```python
from build123d import *

# Parameters (mm, degrees)
SKETCH1_R           = 15
BOSS_EXTRUDE1_DEPTH = 1000
SKETCH2_R           = 20
BOSS_EXTRUDE2_DEPTH = 10
SKETCH3_R           = 15
BOSS_EXTRUDE3_DEPTH = 45
SKETCH4_R           = 20
BOSS_EXTRUDE4_DEPTH = 10
SKETCH5_R           = 15
BOSS_EXTRUDE5_DEPTH = 45


with BuildPart() as part:
    # Sketch1 → Boss-Extrude1 (new body)
    with BuildSketch(Plane.XY):
        Circle(SKETCH1_R)
    extrude(amount=BOSS_EXTRUDE1_DEPTH)

    # Sketch2 → Boss-Extrude2 (add)
    with BuildSketch(Plane.XY.offset(1000)):
        Circle(SKETCH2_R)
    extrude(amount=BOSS_EXTRUDE2_DEPTH)

    # Sketch3 → Boss-Extrude3 (add)
    with BuildSketch(Plane.XY.offset(1010)):
        Circle(SKETCH3_R)
    extrude(amount=BOSS_EXTRUDE3_DEPTH)

    # Sketch4 → Boss-Extrude4 (add)
    with BuildSketch(Plane(origin=(0, 0, 0), x_dir=(-1, 0, 0), z_dir=(0, 0, -1))):
        Circle(SKETCH4_R)
    extrude(amount=BOSS_EXTRUDE4_DEPTH)

    # Sketch5 → Boss-Extrude5 (add)
    with BuildSketch(Plane(origin=(0, 0, -10), x_dir=(-1, 0, 0), z_dir=(0, 0, -1))):
        Circle(SKETCH5_R)
    extrude(amount=BOSS_EXTRUDE5_DEPTH)


solid = part.part
```
Work out the finished part from the listing and answer in its coordinate system (mm). A direction names the side the tool comes from. Give positions to 0.01 mm unless a question says otherwise; leave off trailing zeros. Order: outer loops, then holes, each group sorted by start corner. A loop starts at its lowest first (then second) coordinate and runs counter-clockwise, first axis right, second up. Notation, with made-up numbers: M 13.5,3 L 71.5,3 A18 ccw 71.5,27 Z; hole C 48,40.25 d2. An arc over 180 degrees is marked long. Return JSON: item names as keys, results as strings.
1) For a pull along Z with two mould halves and no side action, classify faces 1 (the cylindrical face through (-14.985, 0.66, 1032.185)), 2 (the flat face through (0, 0, -55)), 3 (the cylindrical face through (-14.985, 0.66, 493)) as +Z half, -Z half, draft (parallel to the pull), parting line (faces both ways), or undercut.
Resolved:
{"face 1": "draft", "face 2": "-Z half", "face 3": "undercut"}
2) Each of these flat-tipped pins is pushed along its axis until it touches: pin 1 (6 mm diameter, centred on y = 0, z = 939, fed in from +X); pin 2 (4 mm diameter, centred on y = -11.5, z = 528.5, fed in from -X); pin 3 (5 mm diameter, centred on x = 3.5, z = 892.5, fed in from +Y). Where does it stop, or does it pass through?
Resolved:
{"pin 1": "x = 15", "pin 2": "x = -11.61", "pin 3": "y = 14.97"}
3) Section C-C, the plane z = 215.5 is taken. Write down the section's boundary in (x, y).
Resolved:
{"outline": "C 0,0 d30"}
4) Straight lines are drawn through the part: line 1 along Z through (x, y) = (-4, 16.5); line 2 along X through (y, z) = (1, 193); line 3 along Y through (x, z) = (-0.5, 739). For each, find the intervals that lie inside material, in ascending order. Write a range as [from, to].
Resolved:
{"line 1": "[-10, 0], [1000, 1010]", "line 2": "[-14.97, 14.97]", "line 3": "[-14.99, 14.99]"}
5) A tool of negligible diameter and unlimited length cuts with its end or side. For faces 4 (the flat face through (3, 15, 1010)), 5 (the flat face through (0, 0, 1055)), 6 (the flat face through (-3, 15, 0)), 7 (the flat face through (-3, 15, -10)), from which of +Z, -Z, +X, -X, +Y, -Y can it reach the whole face along a straight path? Write none if from no direction.
Resolved:
{"face 4": "+Z", "face 5": "+Z, +X, -X, +Y, -Y", "face 6": "none", "face 7": "-Z"}
6) Section A-A, the plane x = 0 is taken. Write down the section's boundary in (y, z).
Resolved:
{"outline": "M -20,-10 L -15,-10 L -15,-55 L 15,-55 L 15,-10 L 20,-10 L 20,0 L 15,0 L 15,1000 L 20,1000 L 20,1010 L 15,1010 L 15,1055 L -15,1055 L -15,1010 L -20,1010 L -20,1000 L -15,1000 L -15,0 L -20,0 Z"}
